```python
from build123d import *

# Parameters (mm, degrees)
SKETCH_1_W          = 155.6
SKETCH_1_H          = 20
SKETCH_1_R          = 4
EXTRUDE_1_DEPTH     = 3
SKETCH_2_W          = 155.6
SKETCH_2_H          = 20
SKETCH_2_W_2        = 149.6
SKETCH_2_H_2        = 14
EXTRUDE_2_DEPTH     = 20
SKETCH_3_R          = 2
CUT_EXTRUDE_1_DEPTH = 160


with BuildPart() as part:
    # 草图1 → 凸台-拉伸1 (new body)
    with BuildSketch(Plane(origin=(0, 0, 0), x_dir=(1, 0, 0), z_dir=(0, 1, 0))):
        Rectangle(SKETCH_1_W, SKETCH_1_H)
        with Locations((-37.5, 0)):
            Circle(SKETCH_1_R, mode=Mode.SUBTRACT)
        with Locations((37.5, 0)):
            Circle(SKETCH_1_R, mode=Mode.SUBTRACT)
    extrude(amount=EXTRUDE_1_DEPTH)

    # 草图2 → 凸台-拉伸2 (add)
    with BuildSketch(Plane(origin=(0, 3, 0), x_dir=(1, 0, 0), z_dir=(0, 1, 0))):
        Rectangle(SKETCH_2_W, SKETCH_2_H)
        Rectangle(SKETCH_2_W_2, SKETCH_2_H_2, mode=Mode.SUBTRACT)
    extrude(amount=EXTRUDE_2_DEPTH)

    # 草图3 → 切除-拉伸1 (cut)
    with BuildSketch(Plane.ZY.offset(77.8)):
        with Locations((0, 13)):
            Circle(SKETCH_3_R)
    extrude(amount=-CUT_EXTRUDE_1_DEPTH, mode=Mode.SUBTRACT)


solid = part.part
```
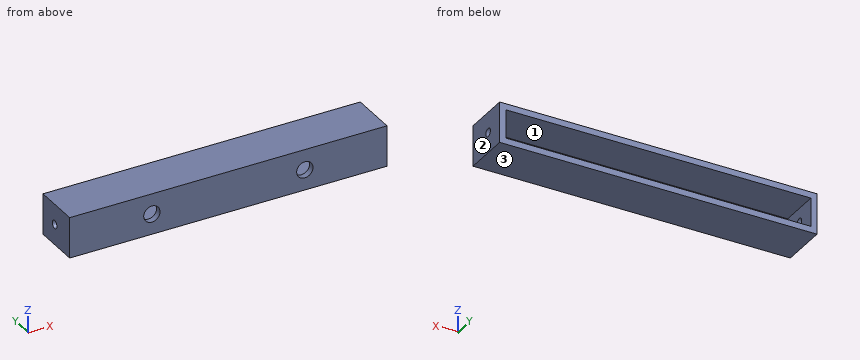
Part model, mm, in its own coordinate system. Face numbers are marked on the shaded views. Round coordinates to 2 decimals unless told otherwise and drop trailing zeros. Loops run counter-clockwise (first coordinate to the right, second up) from the corner with the lowest first, then second, coordinate; pieces in that order, holes last. Notation, with made-up numbers: (-22.5, -4) -> (-2.5, -4) arc R24 ccw to (-2.5, 26) -> close; hole circle Ø2 at (-40, 72). An arc over 180 degrees is marked (long way). Use CSV: the item, a comma, the result in double quotes. Start each with the question number.
1) Wall check: L1, parallel to X at y = 20.25, z = 5.75; L2, parallel to X at y = 1.8, z = 0; L3, parallel to Z at x = 46, y = 17.5. Give the ranges that are in metal, low to high. Write a range as [from, to].
2) Drop a flat-ended pin along its axis: P1, Ø11, axis at x = -29, z = 0.5, coming from the +Y side. Give the stop position or say it passes through.
3) Cut at D-D, the plane y = 13. Write the cut outline in (x, z).
4) Pull direction Z, two halves, no side cores. Call the marked faces 1, 2 and 3: +Z half, -Z half, draft (parallel to the pull), parting line (faces both ways), or undercut.
5) Cut at A-A, the plane z = 0. Write the cut outline in (x, y).
6) Cut at C-C, the plane x = -37.5. Write the cut outline in (y, z), plus the area to 3 significant figures.
7) Cut at B-B, the plane y = 5. Write the cut outline in (x, z).
Determined:
1,L1,"x = [-77.8, -74.8], [74.8, 77.8]"
1,L2,"x = [-77.8, -41.5], [-33.5, 33.5], [41.5, 77.8]"
1,L3,"z = [-10, -7], [7, 10]"
2,P1,"stops at y = 3"
3,outline,"(-77.8, -10) -> (77.8, -10) -> (77.8, -2) -> (74.8, -2) -> (74.8, -7) -> (-74.8, -7) -> (-74.8, -2) -> (-77.8, -2) -> close; (-77.8, 2) -> (-74.8, 2) -> (-74.8, 7) -> (74.8, 7) -> (74.8, 2) -> (77.8, 2) -> (77.8, 10) -> (-77.8, 10) -> close"
4,face 1,"undercut"
4,face 2,"draft"
4,face 3,"-Z half"
5,outline,"(-77.8, 0) -> (-41.5, 0) -> (-41.5, 3) -> (-74.8, 3) -> (-74.8, 11) -> (-77.8, 11) -> close; (-77.8, 15) -> (-74.8, 15) -> (-74.8, 23) -> (-77.8, 23) -> close; (-33.5, 0) -> (33.5, 0) -> (33.5, 3) -> (-33.5, 3) -> close; (41.5, 0) -> (77.8, 0) -> (77.8, 11) -> (74.8, 11) -> (74.8, 3) -> (41.5, 3) -> close; (74.8, 15) -> (77.8, 15) -> (77.8, 23) -> (74.8, 23) -> close"
6,outline,"(0, -10) -> (23, -10) -> (23, -7) -> (3, -7) -> (3, -4) -> (0, -4) -> close; (0, 4) -> (3, 4) -> (3, 7) -> (23, 7) -> (23, 10) -> (0, 10) -> close"
6,area,"156 mm2"
7,outline,"(-77.8, -10) -> (77.8, -10) -> (77.8, 10) -> (-77.8, 10) -> close; hole (-74.8, -7) -> (74.8, -7) -> (74.8, 7) -> (-74.8, 7) -> close"
